Geometry: final body of the model. Coordinates: model frame, mm. Face numbers are marked on the shaded views. A direction names the side the tool comes from. Round coordinates to 2 decimals unless told otherwise and drop trailing zeros. Order: outer loops, then holes, each group sorted by start corner. A loop starts at its lowest first (then second) coordinate and runs counter-clockwise, first axis right, second up. Notation, with made-up numbers: (-0.5, 20.25) - (57.5, 20.25) arc R26 ccw to (57.5, 40.25) - close; hole circle Ø1 at (35, 85.25). An arc over 180 degrees is marked (long way). Put each result on its own line as item: value. Start each with the question number.
(1) Access query for the marked faces 1, 2 and 3. Directions: +Z, -Z, +X, -X, +Y, -Y. A direction counts if a zero-diameter tool reaches every point of the face in a straight line with its end or side. Return the directions, or none.
(2) Section C-C (y = -23.5). Output: boundary loops of the cut face in (x, z).
(3) Section B-B (z = 25). Output: boundary loops of the cut face in (x, y), and give its area (3 significant figures).
(4) Pin query (flat end, axial travel): P1, Ø17.5, axis at y = -20, z = 13, coming from the +X side; P2, Ø1, axis at y = 1.5, z = 20, coming from the +X side; P3, Ø3.5, axis at x = 35.8, z = 20.59, coming from the -Y side. Return the tip coordinate at first contact, or that it passes through.
(5) Section A-A (x = 35.8). Output: boundary loops of the cut face in (y, z).
(6) Section D-D (y = 8.5). Count the separate pieces of the cut face and the enclosed holes in it, and give its area (3 significant figures).
(7) Material intervals for L1, parallel to X at y = 6, z = 5; L2, parallel to X at y = -17, z = 10; L3, parallel to Z at x = 20, y = 6.5, sorted ascending. Write a range as [from, to].
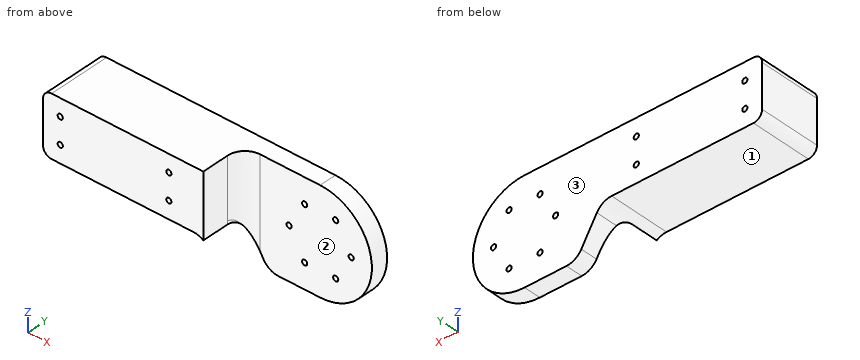
from build123d import *

# Parameters (mm, degrees)
SKETCH1_R           = 1.5
BOSS_EXTRUDE2_DEPTH = 10
BOSS_EXTRUDE3_START = -26
SKETCH1_3_R         = 1.5
BOSS_EXTRUDE3_DEPTH = 26
FILLET1_R           = 10


with BuildPart() as part:
    # Sketch1 → Boss-Extrude2 (new body)
    # profile 1 of 2: a face of its own
    with BuildSketch(Plane(origin=(0, 0, 0), x_dir=(-1, 0, 0), z_dir=(0, 1, 0))):
        with BuildLine():
            Line((0, 35), (-44.8, 35))
            ThreePointArc((-44.8, 35), (-74.8, 5), (-44.8, -25))
            Line((-44.8, -25), (-14.8, -25))
            Line((-14.8, -25), (0, 0))
            Line((0, 0), (0, 35))
        make_face()
        with Locations(Location((-53.8, -10.588457268, 0), (0, 0, 90))):
            Circle(SKETCH1_R, mode=Mode.SUBTRACT)
        with Locations(Location((-35.8, -10.588457268, 0), (0, 0, 90))):
            Circle(SKETCH1_R, mode=Mode.SUBTRACT)
        with Locations(Location((-26.8, 5, 0), (0, 0, 90))):
            Circle(SKETCH1_R, mode=Mode.SUBTRACT)
        with Locations(Location((-35.8, 20.588457268, 0), (0, 0, 90))):
            Circle(SKETCH1_R, mode=Mode.SUBTRACT)
        with Locations(Location((-53.8, 20.588457268, 0), (0, 0, 90))):
            Circle(SKETCH1_R, mode=Mode.SUBTRACT)
        with Locations(Location((-62.8, 5, 0), (0, 0, 90))):
            Circle(SKETCH1_R, mode=Mode.SUBTRACT)
    # profile 2 of 2: a face of its own
    with BuildSketch(Plane(origin=(0, 0, 0), x_dir=(-1, 0, 0), z_dir=(0, 1, 0))):
        with BuildLine():
            ThreePointArc((88, 35), (91.535533906, 33.535533906), (93, 30))
            Line((93, 30), (93, 5))
            ThreePointArc((93, 5), (91.535533906, 1.464466094), (88, 0))
            Line((88, 0), (0, 0))
            Line((0, 0), (0, 35))
            Line((0, 35), (88, 35))
        make_face()
        with Locations(Location((20, 10, 0), (0, 0, 90))):
            Circle(SKETCH1_R, mode=Mode.SUBTRACT)
        with Locations(Location((83, 10, 0), (0, 0, 90))):
            Circle(SKETCH1_R, mode=Mode.SUBTRACT)
        with Locations(Location((83, 25, 0), (0, 0, 90))):
            Circle(SKETCH1_R, mode=Mode.SUBTRACT)
        with Locations(Location((20, 25, 0), (0, 0, 90))):
            Circle(SKETCH1_R, mode=Mode.SUBTRACT)
    extrude(amount=BOSS_EXTRUDE2_DEPTH)

    # Sketch1<3> → Boss-Extrude3 (add)
    with BuildSketch(Plane(origin=(0, 0, 0), x_dir=(-1, 0, 0), z_dir=(0, 1, 0)).offset(BOSS_EXTRUDE3_START)):
        with BuildLine():
            ThreePointArc((88, 35), (91.535533906, 33.535533906), (93, 30))
            Line((93, 30), (93, 5))
            ThreePointArc((93, 5), (91.535533906, 1.464466094), (88, 0))
            Line((88, 0), (0, 0))
            Line((0, 0), (0, 35))
            Line((0, 35), (88, 35))
        make_face()
        with Locations(Location((20, 10, 0), (0, 0, 90))):
            Circle(SKETCH1_3_R, mode=Mode.SUBTRACT)
        with Locations(Location((83, 10, 0), (0, 0, 90))):
            Circle(SKETCH1_3_R, mode=Mode.SUBTRACT)
        with Locations(Location((83, 25, 0), (0, 0, 90))):
            Circle(SKETCH1_3_R, mode=Mode.SUBTRACT)
        with Locations(Location((20, 25, 0), (0, 0, 90))):
            Circle(SKETCH1_3_R, mode=Mode.SUBTRACT)
    extrude(amount=BOSS_EXTRUDE3_DEPTH)

    # Fillet1
    # the kernel refuses this fillet: 10 mm, written as the material it adds along each edge
    with BuildSketch(Plane(origin=(0, 0, -60), x_dir=(0, -1, 0), z_dir=(0, 0, 1))) as fillet1_piece_1_section:
        with BuildLine():
            CenterArc((FILLET1_R, FILLET1_R), FILLET1_R, 180, 90)
            Line((0, FILLET1_R), (-FILLET1_R * 0.02, FILLET1_R))
            Line((-FILLET1_R * 0.02, FILLET1_R), (-FILLET1_R * 0.02, -FILLET1_R * 0.02))
            Line((-FILLET1_R * 0.02, -FILLET1_R * 0.02), (FILLET1_R, -FILLET1_R * 0.02))
            Line((FILLET1_R, -FILLET1_R * 0.02), (FILLET1_R, 0))
        make_face()
    fillet1_piece_1 = extrude(amount=95, mode=Mode.PRIVATE)
    fillet1_piece_1 = split(fillet1_piece_1, bisect_by=Plane(origin=(4.301180518, -1.064725153, 0), z_dir=(0, 0, -1)), keep=Keep.TOP, mode=Mode.PRIVATE)
    fillet1_piece_1 = split(fillet1_piece_1, bisect_by=Plane(origin=(2.708698038, -1.064725153, -4.575503443), z_dir=(0.8605150974154716, 0, 0.509424937669959)), keep=Keep.TOP, mode=Mode.PRIVATE)
    add(fillet1_piece_1)
    with BuildSketch(Plane(origin=(0, 0, 0), x_dir=(0, -1, 0), z_dir=(0, 0, 1))) as fillet1_piece_2_section:
        with BuildLine():
            CenterArc((FILLET1_R, FILLET1_R), FILLET1_R, 180, 90)
            Line((0, FILLET1_R), (-FILLET1_R * 0.02, FILLET1_R))
            Line((-FILLET1_R * 0.02, FILLET1_R), (-FILLET1_R * 0.02, -FILLET1_R * 0.02))
            Line((-FILLET1_R * 0.02, -FILLET1_R * 0.02), (FILLET1_R, -FILLET1_R * 0.02))
            Line((FILLET1_R, -FILLET1_R * 0.02), (FILLET1_R, 0))
        make_face()
    fillet1_piece_2 = extrude(amount=35, mode=Mode.PRIVATE)
    fillet1_piece_2 = split(fillet1_piece_2, bisect_by=Plane(origin=(-7.086614588, -2.262932977, 11.97063275), z_dir=(0.8605150974154716, 0, 0.509424937669959)), keep=Keep.TOP, mode=Mode.PRIVATE)
    add(fillet1_piece_2)
    with BuildSketch(Plane(origin=(0, 0, 0), x_dir=(0, -1, 0), z_dir=(0, 0, 1))) as fillet1_piece_3_section:
        with BuildLine():
            CenterArc((FILLET1_R, FILLET1_R), FILLET1_R, 180, 90)
            Line((0, FILLET1_R), (-FILLET1_R * 0.02, FILLET1_R))
            Line((-FILLET1_R * 0.02, FILLET1_R), (-FILLET1_R * 0.02, -FILLET1_R * 0.02))
            Line((-FILLET1_R * 0.02, -FILLET1_R * 0.02), (FILLET1_R, -FILLET1_R * 0.02))
            Line((FILLET1_R, -FILLET1_R * 0.02), (FILLET1_R, 0))
        make_face()
    fillet1_piece_3 = extrude(amount=35, mode=Mode.PRIVATE)
    fillet1_piece_3 = split(fillet1_piece_3, bisect_by=Plane(origin=(-0.083967584, -4.9, 0.141837136), z_dir=(-0.8605150974154716, 0, -0.509424937669959)), keep=Keep.TOP, mode=Mode.PRIVATE)
    add(fillet1_piece_3)
    with BuildSketch(Plane(origin=(0, -34.205679631, 0), x_dir=(-1, 0, 0), z_dir=(0, 1, 0))) as fillet1_piece_4_section:
        with BuildLine():
            CenterArc((FILLET1_R * 0.570094660516, -FILLET1_R), FILLET1_R, 90, 59.374467281)
            Line((-FILLET1_R * 0.290420436899, -FILLET1_R * 0.49057506233), (-FILLET1_R * 0.307630738848, -FILLET1_R * 0.480386563577))
            Line((-FILLET1_R * 0.307630738848, -FILLET1_R * 0.480386563577), (-FILLET1_R * 0.0114018932103, FILLET1_R * 0.02))
            Line((-FILLET1_R * 0.0114018932103, FILLET1_R * 0.02), (FILLET1_R * 0.570094660516, FILLET1_R * 0.02))
            Line((FILLET1_R * 0.570094660516, FILLET1_R * 0.02), (FILLET1_R * 0.570094660516, 0))
        make_face()
    fillet1_piece_4 = extrude(amount=44.205679631, mode=Mode.PRIVATE)
    fillet1_piece_4 = split(fillet1_piece_4, bisect_by=Plane(origin=(0, -13, -0.363733484), z_dir=(-1, 0, 0)), keep=Keep.TOP, mode=Mode.PRIVATE)
    fillet1_piece_4 = split(fillet1_piece_4, bisect_by=Plane(origin=(-1.77482193, -26, -0.363733484), z_dir=(0, 1, 0)), keep=Keep.TOP, mode=Mode.PRIVATE)
    fillet1_piece_4 = split(fillet1_piece_4, bisect_by=Plane(origin=(-1.77482193, 0, -0.363733484), z_dir=(0, -1, 0)), keep=Keep.TOP, mode=Mode.PRIVATE)
    add(fillet1_piece_4)
    with BuildSketch(Plane(origin=(0, 0, 0), x_dir=(-1, 0, 0), z_dir=(0, 1, 0))) as fillet1_piece_5_section:
        with BuildLine():
            CenterArc((FILLET1_R * 0.570094660516, -FILLET1_R), FILLET1_R, 90, 59.374467281)
            Line((-FILLET1_R * 0.290420436899, -FILLET1_R * 0.49057506233), (-FILLET1_R * 0.307630738848, -FILLET1_R * 0.480386563577))
            Line((-FILLET1_R * 0.307630738848, -FILLET1_R * 0.480386563577), (-FILLET1_R * 0.0114018932103, FILLET1_R * 0.02))
            Line((-FILLET1_R * 0.0114018932103, FILLET1_R * 0.02), (FILLET1_R * 0.570094660516, FILLET1_R * 0.02))
            Line((FILLET1_R * 0.570094660516, FILLET1_R * 0.02), (FILLET1_R * 0.570094660516, 0))
        make_face()
    fillet1_piece_5 = extrude(amount=10, mode=Mode.PRIVATE)
    fillet1_piece_5 = split(fillet1_piece_5, bisect_by=Plane(origin=(0, 5, -0.363733484), z_dir=(-1, 0, 0)), keep=Keep.TOP, mode=Mode.PRIVATE)
    add(fillet1_piece_5)
    with BuildSketch(Plane(origin=(0, 0, 0), x_dir=(-1, 0, 0), z_dir=(0, 1, 0))) as fillet1_piece_6_section:
        with BuildLine():
            CenterArc((FILLET1_R * 0.570094660516, -FILLET1_R), FILLET1_R, 90, 59.374467281)
            Line((-FILLET1_R * 0.290420436899, -FILLET1_R * 0.49057506233), (-FILLET1_R * 0.307630738848, -FILLET1_R * 0.480386563577))
            Line((-FILLET1_R * 0.307630738848, -FILLET1_R * 0.480386563577), (-FILLET1_R * 0.0114018932103, FILLET1_R * 0.02))
            Line((-FILLET1_R * 0.0114018932103, FILLET1_R * 0.02), (FILLET1_R * 0.570094660516, FILLET1_R * 0.02))
            Line((FILLET1_R * 0.570094660516, FILLET1_R * 0.02), (FILLET1_R * 0.570094660516, 0))
        make_face()
    fillet1_piece_6 = extrude(amount=10, mode=Mode.PRIVATE)
    fillet1_piece_6 = split(fillet1_piece_6, bisect_by=Plane(origin=(0, 5, -2.053594733), z_dir=(1, 0, 0)), keep=Keep.TOP, mode=Mode.PRIVATE)
    add(fillet1_piece_6)
    with BuildSketch(Plane(origin=(0, -34.205679631, 0), x_dir=(-1, 0, 0), z_dir=(0, 1, 0))) as fillet1_piece_7a_section:
        with BuildLine():
            CenterArc((FILLET1_R * 0.570094660516, -FILLET1_R), FILLET1_R, 90, 59.374467281)
            Line((-FILLET1_R * 0.290420436899, -FILLET1_R * 0.49057506233), (-FILLET1_R * 0.307630738848, -FILLET1_R * 0.480386563577))
            Line((-FILLET1_R * 0.307630738848, -FILLET1_R * 0.480386563577), (-FILLET1_R * 0.0114018932103, FILLET1_R * 0.02))
            Line((-FILLET1_R * 0.0114018932103, FILLET1_R * 0.02), (FILLET1_R * 0.570094660516, FILLET1_R * 0.02))
            Line((FILLET1_R * 0.570094660516, FILLET1_R * 0.02), (FILLET1_R * 0.570094660516, 0))
        make_face()
    fillet1_piece_7a = extrude(amount=44.205679631, mode=Mode.PRIVATE)
    fillet1_piece_7a = split(fillet1_piece_7a, bisect_by=Plane(origin=(0, -13, -2.053594733), z_dir=(1, 0, 0)), keep=Keep.TOP, mode=Mode.PRIVATE)
    fillet1_piece_7a = split(fillet1_piece_7a, bisect_by=Plane(origin=(1.054652956, -26, -2.053594733), z_dir=(0, 1, 0)), keep=Keep.TOP, mode=Mode.PRIVATE)
    fillet1_piece_7a = split(fillet1_piece_7a, bisect_by=Plane(origin=(1.054652956, 0, -2.053594733), z_dir=(0, -1, 0)), keep=Keep.TOP, mode=Mode.PRIVATE)
    with BuildSketch(Plane(origin=(0, 0, -60), x_dir=(0, -1, 0), z_dir=(0, 0, 1))) as fillet1_piece_7b_section:
        with BuildLine():
            CenterArc((FILLET1_R, FILLET1_R), FILLET1_R, 180, 90)
            Line((0, FILLET1_R), (-FILLET1_R * 0.02, FILLET1_R))
            Line((-FILLET1_R * 0.02, FILLET1_R), (-FILLET1_R * 0.02, -FILLET1_R * 0.02))
            Line((-FILLET1_R * 0.02, -FILLET1_R * 0.02), (FILLET1_R, -FILLET1_R * 0.02))
            Line((FILLET1_R, -FILLET1_R * 0.02), (FILLET1_R, 0))
        make_face()
    fillet1_piece_7b = extrude(amount=95, mode=Mode.PRIVATE)
    fillet1_piece_7b = split(fillet1_piece_7b, bisect_by=Plane(origin=(2.124740403, -2.345898291, 0), z_dir=(0, 0, -1)), keep=Keep.TOP, mode=Mode.PRIVATE)
    fillet1_piece_7b = split(fillet1_piece_7b, bisect_by=Plane(origin=(14.492269712, -2.345898291, -24.480185325), z_dir=(-0.8605150974154716, 0, -0.509424937669959)), keep=Keep.TOP, mode=Mode.PRIVATE)
    fillet1_piece_7 = fillet1_piece_7a & fillet1_piece_7b
    add(fillet1_piece_7)
    # the kernel refuses this fillet: 10 mm, written as the material it takes off along each edge
    with BuildSketch(Plane(origin=(14.8, -34.205679631, -25), x_dir=(-0.5094249376699589, 0, 0.8605150974154715), z_dir=(0, 1, 0))) as fillet1_2_piece_1:
        with BuildLine():
            CenterArc((FILLET1_R * 0.570094660516, FILLET1_R), FILLET1_R, 210.625532719, 59.374467281)
            Line((-FILLET1_R * 0.290420436899, FILLET1_R * 0.49057506233), (-FILLET1_R * 0.307630738848, FILLET1_R * 0.480386563577))
            Line((-FILLET1_R * 0.307630738848, FILLET1_R * 0.480386563577), (-FILLET1_R * 0.0114018932103, -FILLET1_R * 0.02))
            Line((-FILLET1_R * 0.0114018932103, -FILLET1_R * 0.02), (FILLET1_R * 0.570094660516, -FILLET1_R * 0.02))
            Line((FILLET1_R * 0.570094660516, -FILLET1_R * 0.02), (FILLET1_R * 0.570094660516, 0))
        make_face()
    extrude(amount=78.411359262, mode=Mode.SUBTRACT)


solid = part.part
Checks:
1. face 1: -Z, -X, +Y, -Y
1. face 2: +Z, -Z, +X, -Y
1. face 3: +Z, -Z, +X, -X, +Y
2. outline: (-93, 5) arc R5 ccw to (-88, 0) - (-5.7, 0) arc R10 cw to (0, -1.78) - (0, 35) - (-88, 35) arc R5 ccw to (-93, 30) - close; hole circle Ø3 at (-83, 10); hole circle Ø3 at (-83, 25); hole circle Ø3 at (-20, 10); hole circle Ø3 at (-20, 25)
3. outline: (-93, -26) - (-84.5, -26) - (-84.5, 10) - (-93, 10) - close; (-81.5, -26) - (-21.5, -26) - (-21.5, 10) - (-81.5, 10) - close; (-18.5, -26) - (0, -26) - (0, -10) arc R10 cw to (10, 0) - (67.16, 0) - (67.16, 10) - (-18.5, 10) - close
3. area: 3,830 mm²
4. P1: stops at x = 0
4. P2: stops at x = 71.06
4. P3: stops at y = 0
5. outline: (0, -25) - (10, -25) - (10, -12.09) - (0, -12.09) - close; (0, -9.09) - (10, -9.09) - (10, 19.09) - (0, 19.09) - close; (0, 22.09) - (10, 22.09) - (10, 35) - (0, 35) - close
6. separate pieces: 1
6. enclosed holes: 10
6. area: 7,090 mm²
7. L1: x = [-93, 25.3], [28.3, 61.3], [64.3, 74.8]
7. L2: x = [-93, -84.5], [-81.5, -21.5], [-18.5, 0]
7. L3: z = [-24.99, 35]
